from build123d import *

# Parameters (mm, degrees)
F0_R         = 12.65
F1_DEPTH     = 26
F2_W         = 14
F2_H         = 29.3698692877
F3_DEPTH     = 16
F4_T1_DEPTH  = 21.3868200642
F4_T6_ANGLE  = 89.8472397972
F4_T12_ANGLE = 89.8472397972
F4_T19_DEPTH = 26.7736401284
F4_T23_ANGLE = 89.8472397972
F4_T30_ANGLE = 89.8472397972
F4_T34_DEPTH = 26.7736401284
F4_T41_ANGLE = 89.8472397972
F4_T45_DEPTH = 26.7736401284
F4_T52_DEPTH = 26.7736401284
F4_T56_ANGLE = 89.8472397972
F5_R         = 4
F6_DEPTH     = 16.2


# Not quite as in the source:
# - a fillet or chamfer that OpenCascade refuses, or shapes differently, is made with other operations: its cross-section is extruded or revolved along the edge and cut away or added


with BuildPart() as f1:
    # F0 (on Top) → F1 (new body)
    with BuildSketch(Plane.XY):
        Circle(F0_R)
    extrude(amount=F1_DEPTH)

    # F2 (on Top) → F3 (cut)
    with BuildSketch(Plane.XY):
        Rectangle(F2_W, F2_H)
    extrude(amount=F3_DEPTH, mode=Mode.SUBTRACT)

    # F4: fillet of radius 1 on 6 edges, made by hand

    # F4_s2 → F4_t1 (cut)
    with BuildSketch(Plane.XY.offset(-5.3868200642)):
        with BuildLine():
            ThreePointArc((8.686695279, 9.1958591295), (7.6042066694, 9.3872533539), (7, 8.4689137438))
            Line((7, 8.4689137438), (7, 10.5367215015))
            ThreePointArc((7, 10.5367215015), (7.8719489435, 9.9022684185), (8.686695279, 9.1958591295))
        make_face()
        with BuildLine():
            ThreePointArc((8.686695279, -9.1958591295), (7.6042066694, -9.3872533539), (7, -8.4689137438))
            Line((7, -8.4689137438), (7, -10.5367215015))
            ThreePointArc((7, -10.5367215015), (7.8719489435, -9.9022684185), (8.686695279, -9.1958591295))
        make_face()
        with BuildLine():
            ThreePointArc((-8.686695279, 9.1958591295), (-7.6042066694, 9.3872533539), (-7, 8.4689137438))
            Line((-7, 8.4689137438), (-7, 10.5367215015))
            ThreePointArc((-7, 10.5367215015), (-7.8719489435, 9.9022684185), (-8.686695279, 9.1958591295))
        make_face()
        with BuildLine():
            ThreePointArc((-8.686695279, -9.1958591295), (-7.6042066694, -9.3872533539), (-7, -8.4689137438))
            Line((-7, -8.4689137438), (-7, -10.5367215015))
            ThreePointArc((-7, -10.5367215015), (-7.8719489435, -9.9022684185), (-8.686695279, -9.1958591295))
        make_face()
    extrude(amount=F4_T1_DEPTH, mode=Mode.SUBTRACT)


with BuildPart() as f4_tool4:
    # F4_s5 → F4_t6 (revolve)
    with BuildSketch(Plane(origin=(0, 0, 0), x_dir=(0, 0, 1), z_dir=(-0.7080487855, -0.7061635202, 0))):
        with BuildLine():
            ThreePointArc((17, 12.65), (16.2928932188, 12.3571067812), (16, 11.65))
            Line((16, 11.65), (16, 12.65))
            Line((16, 12.65), (17, 12.65))
        make_face()
    revolve(axis=Axis((0, 0, 16), (0, 0, -1)), revolution_arc=F4_T6_ANGLE)

    split(bisect_by=Plane.YZ.offset(7), keep=Keep.BOTTOM)

    split(bisect_by=Plane.YZ.offset(-7), keep=Keep.TOP)


with BuildPart() as f1_1:
    add(f1.part)

    # F4_t3: cut F4_tool4
    add(f4_tool4.part, mode=Mode.SUBTRACT)


with BuildPart() as f4_tool10:
    # F4_s11 → F4_t12 (revolve)
    with BuildSketch(Plane(origin=(0, 0, 0), x_dir=(0, 0, 1), z_dir=(0.7080487855, 0.7061635202, 0))):
        with BuildLine():
            ThreePointArc((17, 12.65), (16.2928932188, 12.3571067812), (16, 11.65))
            Line((16, 11.65), (16, 12.65))
            Line((16, 12.65), (17, 12.65))
        make_face()
    revolve(axis=Axis((0, 0, 16), (0, 0, -1)), revolution_arc=F4_T12_ANGLE)

    split(bisect_by=Plane.YZ.offset(7), keep=Keep.BOTTOM)

    split(bisect_by=Plane.YZ.offset(-7), keep=Keep.TOP)


with BuildPart() as f1_2:
    add(f1_1.part)

    # F4_t9: cut F4_tool10
    add(f4_tool10.part, mode=Mode.SUBTRACT)


with BuildPart() as f4_tool17:
    # F4_s18 → F4_t19 (new body)
    with BuildSketch(Plane.XY.offset(21.3868200642)):
        with BuildLine():
            ThreePointArc((8.686695279, 9.1958591295), (7.6042066694, 9.3872533539), (7, 8.4689137438))
            Line((7, 8.4689137438), (7, 10.5367215015))
            ThreePointArc((7, 10.5367215015), (7.8719489435, 9.9022684185), (8.686695279, 9.1958591295))
        make_face()
    extrude(amount=-F4_T19_DEPTH)

    split(bisect_by=Plane.XY.offset(16), keep=Keep.TOP)


with BuildPart() as f4_tool21:
    # F4_s22 → F4_t23 (revolve)
    with BuildSketch(Plane(origin=(0, 0, 0), x_dir=(0, 0, 1), z_dir=(-0.7080487855, -0.7061635202, 0))):
        with BuildLine():
            ThreePointArc((17, 12.65), (16.2928932188, 12.3571067812), (16, 11.65))
            Line((16, 11.65), (16, 12.65))
            Line((16, 12.65), (17, 12.65))
        make_face()
    revolve(axis=Axis((0, 0, 16), (0, 0, -1)), revolution_arc=F4_T23_ANGLE)

    split(bisect_by=Plane.YZ.offset(7), keep=Keep.TOP)


with BuildPart() as f4_tool17_1:
    add(f4_tool17.part)

    # F4_t25: intersect F4_tool21
    add(f4_tool21.part, mode=Mode.INTERSECT)


with BuildPart() as f1_3:
    add(f1_2.part)

    # F4_t15: cut F4_tool17
    add(f4_tool17_1.part, mode=Mode.SUBTRACT)


with BuildPart() as f4_tool28:
    # F4_s29 → F4_t30 (revolve)
    with BuildSketch(Plane(origin=(0, 0, 0), x_dir=(0, 0, 1), z_dir=(0.7080487855, 0.7061635202, 0))):
        with BuildLine():
            ThreePointArc((17, 12.65), (16.2928932188, 12.3571067812), (16, 11.65))
            Line((16, 11.65), (16, 12.65))
            Line((16, 12.65), (17, 12.65))
        make_face()
    revolve(axis=Axis((0, 0, 16), (0, 0, -1)), revolution_arc=F4_T30_ANGLE)

    split(bisect_by=Plane.YZ.offset(7), keep=Keep.TOP)


with BuildPart() as f4_tool32:
    # F4_s33 → F4_t34 (new body)
    with BuildSketch(Plane.XY.offset(21.3868200642)):
        with BuildLine():
            ThreePointArc((8.686695279, -9.1958591295), (7.6042066694, -9.3872533539), (7, -8.4689137438))
            Line((7, -8.4689137438), (7, -10.5367215015))
            ThreePointArc((7, -10.5367215015), (7.8719489435, -9.9022684185), (8.686695279, -9.1958591295))
        make_face()
    extrude(amount=-F4_T34_DEPTH)

    split(bisect_by=Plane.XY.offset(16), keep=Keep.TOP)


with BuildPart() as f4_tool28_1:
    add(f4_tool28.part)

    # F4_t36: intersect F4_tool32
    add(f4_tool32.part, mode=Mode.INTERSECT)


with BuildPart() as f1_4:
    add(f1_3.part)

    # F4_t26: cut F4_tool28
    add(f4_tool28_1.part, mode=Mode.SUBTRACT)


with BuildPart() as f4_tool39:
    # F4_s40 → F4_t41 (revolve)
    with BuildSketch(Plane(origin=(0, 0, 0), x_dir=(0, 0, 1), z_dir=(-0.7080487855, -0.7061635202, 0))):
        with BuildLine():
            ThreePointArc((17, 12.65), (16.2928932188, 12.3571067812), (16, 11.65))
            Line((16, 11.65), (16, 12.65))
            Line((16, 12.65), (17, 12.65))
        make_face()
    revolve(axis=Axis((0, 0, 16), (0, 0, -1)), revolution_arc=F4_T41_ANGLE)

    split(bisect_by=Plane.YZ.offset(-7), keep=Keep.BOTTOM)


with BuildPart() as f4_tool43:
    # F4_s44 → F4_t45 (new body)
    with BuildSketch(Plane.XY.offset(21.3868200642)):
        with BuildLine():
            ThreePointArc((-8.686695279, 9.1958591295), (-7.6042066694, 9.3872533539), (-7, 8.4689137438))
            Line((-7, 8.4689137438), (-7, 10.5367215015))
            ThreePointArc((-7, 10.5367215015), (-7.8719489435, 9.9022684185), (-8.686695279, 9.1958591295))
        make_face()
    extrude(amount=-F4_T45_DEPTH)

    split(bisect_by=Plane.XY.offset(16), keep=Keep.TOP)


with BuildPart() as f4_tool39_1:
    add(f4_tool39.part)

    # F4_t47: intersect F4_tool43
    add(f4_tool43.part, mode=Mode.INTERSECT)


with BuildPart() as f1_5:
    add(f1_4.part)

    # F4_t37: cut F4_tool39
    add(f4_tool39_1.part, mode=Mode.SUBTRACT)


with BuildPart() as f4_tool50:
    # F4_s51 → F4_t52 (new body)
    with BuildSketch(Plane.XY.offset(21.3868200642)):
        with BuildLine():
            ThreePointArc((-8.686695279, -9.1958591295), (-7.6042066694, -9.3872533539), (-7, -8.4689137438))
            Line((-7, -8.4689137438), (-7, -10.5367215015))
            ThreePointArc((-7, -10.5367215015), (-7.8719489435, -9.9022684185), (-8.686695279, -9.1958591295))
        make_face()
    extrude(amount=-F4_T52_DEPTH)

    split(bisect_by=Plane.XY.offset(16), keep=Keep.TOP)


with BuildPart() as f4_tool54:
    # F4_s55 → F4_t56 (revolve)
    with BuildSketch(Plane(origin=(0, 0, 0), x_dir=(0, 0, 1), z_dir=(0.7080487855, 0.7061635202, 0))):
        with BuildLine():
            ThreePointArc((17, 12.65), (16.2928932188, 12.3571067812), (16, 11.65))
            Line((16, 11.65), (16, 12.65))
            Line((16, 12.65), (17, 12.65))
        make_face()
    revolve(axis=Axis((0, 0, 16), (0, 0, -1)), revolution_arc=F4_T56_ANGLE)

    split(bisect_by=Plane.YZ.offset(-7), keep=Keep.BOTTOM)


with BuildPart() as f4_tool50_1:
    add(f4_tool50.part)

    # F4_t58: intersect F4_tool54
    add(f4_tool54.part, mode=Mode.INTERSECT)


with BuildPart() as f1_6:
    add(f1_5.part)

    # F4_t48: cut F4_tool50
    add(f4_tool50_1.part, mode=Mode.SUBTRACT)

    # F5 (on Right) → F6 (cut, symmetric)
    with BuildSketch(Plane.YZ):
        with Locations((0, 8)):
            Circle(F5_R)
    extrude(amount=F6_DEPTH, both=True, mode=Mode.SUBTRACT)


solid = f1_6.part
The listing builds one solid part. Answer for the finished solid, in the listing's coordinates (mm). A direction names the side the tool comes from. Round coordinates to 2 decimals unless told otherwise and drop trailing zeros. Order: outer loops, then holes, each group sorted by start corner. A loop starts at its lowest first (then second) coordinate and runs counter-clockwise, first axis right, second up. Notation, with made-up numbers: (31, 59) - (87, 59) arc R36 cw to (87, 93) - close; hole circle Ø4 at (-26.5, 74.5). An arc over 180 degrees is marked (long way). Write item = value, one per line. Start each with the question number.
1) Section C-C, the plane x = 0 is taken. Write down the section's boundary in (y, z), plus the area to 3 significant figures.
2) Section B-B, the plane z = 8 is taken. Write down the section's boundary in (x, y), plus the area to 3 significant figures.
3) Straight lines are drawn through the part: L1, parallel to Z at x = -11.3, y = 0; L2, parallel to Z at x = 4.75, y = 6.5; L3, parallel to Y at x = 9.1, z = 8. For each, find the intervals that lie inside material, in ascending order.
4) For a pull along Y with two mould halves and no side action, classify faces 1 (the cylindrical face through (-12.638, 0.556, 15.707)), 2 (the cylindrical face through (-9.785, -0.521, 11.966)), 3 (the flat face through (7, 2, 4)), 4 (the cylindrical face through (9.865, 3.695, 6.468)) as released by +Y, released by -Y, zero draft, split by the parting line, or undercut.
5) For faces 5 (the flat face through (-7, 2, 4)), 6 (the cylindrical face through (7.619, 9.394, 8.381)), 7 (the cylindrical face through (-7.619, -9.394, 8.381)), determine the directions among +Z, -Z, +X, -X, +Y, -Y from which every point of the face is accessible in a straight line to the end or side of a thin tool.
6) Given pin 1 (12 mm diameter, centred on x = 6.5, z = 18.5, fed in from +Y); pin 2 (7 mm diameter, centred on x = 1, y = 5, fed in from -Z); pin 3 (5 mm diameter, centred on y = 2.5, z = 6, fed in from -X), each flat-ended and moving along its own axis, determine where each tip first touches the part or whether it passes through.
7) Section D-D, the plane z = 14.5 is taken. Write down the section's boundary in (x, y).
8) Section A-A, the plane y = 0 is taken. Write down the section's boundary in (x, z), plus the area to 3 significant figures.
Results list:
q1.outline = (-12.65, 17) arc R1 ccw to (-11.65, 16) - (11.65, 16) arc R1 ccw to (12.65, 17) - (12.65, 26) - (-12.65, 26) - close
q1.area = 253 mm^2
q2.outline = (-12, -4) arc R12.65 ccw to (-8.69, -9.2) arc R1 ccw to (-7, -8.47) - (-7, -4) - close; (-12, 4) - (-7, 4) - (-7, 8.47) arc R1 ccw to (-8.69, 9.2) arc R12.65 ccw to start; (7, -8.47) arc R1 ccw to (8.69, -9.2) arc R12.65 ccw to (12, -4) - (7, -4) - close; (7, 4) - (12, 4) arc R12.65 ccw to (8.69, 9.2) arc R1 ccw to (7, 8.47) - close
q2.area = 76.5 mm^2
q3.L1 = 0 to 4, 12 to 26
q3.L2 = 16 to 26
q3.L3 = -8.79 to -4, 4 to 8.79
q4.face_1 = split by the parting line
q4.face_2 = undercut
q4.face_3 = zero draft
q4.face_4 = undercut
q5.face_5 = -Z, +Y, -Y
q5.face_6 = -Z, +Y
q5.face_7 = -Z, -Y
q6.pin_1 = 12.64
q6.pin_2 = 16
q6.pin_3 = -12.62
q7.outline = (-8.69, -9.2) arc R1 ccw to (-7, -8.47) - (-7, 8.47) arc R1 ccw to (-8.69, 9.2) arc R12.65 ccw to start; (7, -8.47) arc R1 ccw to (8.69, -9.2) arc R12.65 ccw to (8.69, 9.2) arc R1 ccw to (7, 8.47) - close
q8.outline = (-12.65, 0) - (-7, 0) - (-7, 4) - (-12.65, 4) - close; (-12.65, 12) - (-7, 12) - (-7, 16) - (7, 16) - (7, 12) - (12.65, 12) - (12.65, 26) - (-12.65, 26) - close; (7, 0) - (12.65, 0) - (12.65, 4) - (7, 4) - close
q8.area = 343 mm^2
